Source: CAD feature listing. Evaluate the final solid. Frame: model axes, mm. Round coordinates to 2 decimals unless told otherwise and drop trailing zeros. Order: outer loops, then holes, each group sorted by start corner. A loop starts at its lowest first (then second) coordinate and runs counter-clockwise, first axis right, second up. Notation, with made-up numbers: M 44.5,20.5 L 75.5,20.5 A19 cw 75.5,44.5 Z; hole C 56.5,6.25 d5. An arc over 180 degrees is marked long. Use one line per item in the form item = value. Start each with the question number.
Q1. Section A-A (x = -29.5). Return the cut outline in (y, z), plus the area to 3 significant figures.
Q2. Contact query for a flat-ended pin moving along its axis: pin 1 (1.5 mm diameter, centred on y = 3, z = -2.5, fed in from +X). Output: stop coordinate, or through.
Q3. Material intervals for probe 1 along Y at (x, z) = (-2.65, -2.5); probe 2 along Z at (x, y) = (-1.45, 3); probe 3 along X at (y, z) = (2.9, -0.55), sorted ascending.
Q4. Section B-B (x = -4). Return the cut outline in (y, z), plus the area to 3 significant figures.
Autodesk Inventor part; units mm, degrees
ref_plane "作業平面1" through (-29.5, 0, 0) normal (1, 0, 0) x (0, 0, -1)
ref_plane "YZ Plane" through (0, 0, 0) normal (1, 0, 0) x (0, 1, 0)
ref_plane "XZ Plane" through (0, 0, 0) normal (0, 1, 0) x (-1, 0, 0)
sketch "スケッチ1" plane through (0, 0, 0) normal (1, 0, 0) x (0, 1, 0)
  line L0 (0, 0) -> (6, 0)
  line L1 (6, 0) -> (6, -5)
  line L2 (6, -5) -> (0, -5)
  line L3 (0, -5) -> (0, 0)
  point P0 (3, -2.5)
  dimension "d0" = 6
  dimension "d1" = 5
  dimension "d2" = 3
  dimension "d3" = 2.5
extrude "押し出し1" add sketch "スケッチ1" against normal blind 59
ref_plane "作業平面1" through (-29.5, 0, 0) normal (1, 0, 0) x (0, 0, -1)
hole "穴1" at (0, 3, -2.5) direction (-1, 0, 0) diameter 2.5 depth 5 tip angle 118
mirror "ミラー1" about plane through (-29.5, 0, 0) normal (1, 0, 0) of "穴1"
sketch "スケッチ2" plane through (0, 0, 0) normal (0, 0, 1) x (1, 0, 0)
  circle A0 centre (-29.5, 3) radius 1.25
  line L0 (0, 6) -> (-59, 6)
  line L1 (0, 6) -> (0, 0)
  dimension "d14" = 2.5
  dimension "d15" = 3
  dimension "d16" = 29.5
extrude "押し出し2" cut sketch "スケッチ2" against normal blind 59
properties part number "belt_liner_v2_Plate_7" material "アルミニウム 6061"
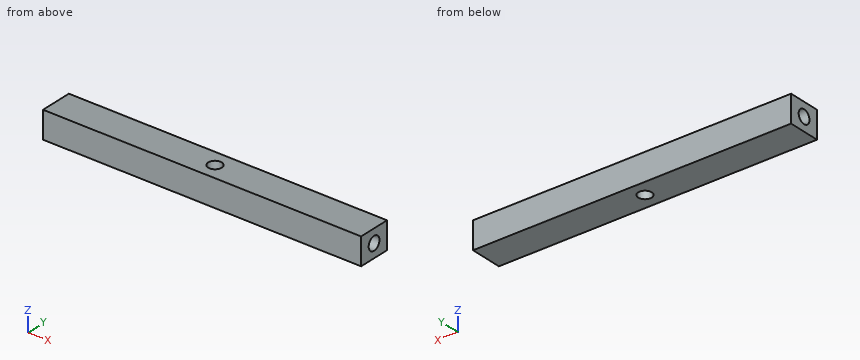
Results list:
q1.outline = M 0,-5 L 1.75,-5 L 1.75,0 L 0,0 Z; M 4.25,-5 L 6,-5 L 6,0 L 4.25,0 Z
q1.area = 17.5 mm2
q2.pin_1 = -5.3
q3.probe_1 = 0 to 1.75, 4.25 to 6
q3.probe_2 = -5 to -3.75, -1.25 to 0
q3.probe_3 = -59 to -30.75, -28.25 to 0
q4.outline = M 0,-5 L 6,-5 L 6,0 L 0,0 Z; hole C 3,-2.5 d2.5
q4.area = 25.1 mm2
